from build123d import *

# Parameters (mm, degrees)
F0_W     = 3.175
F0_H     = 28.575
F1_DEPTH = 15.875
F2_R     = 3.175
F3_R     = 5.08
F4_R     = 4.7625
F5_DEPTH = 3.176
F6_W     = 4.7625
F6_H     = 11.1125
F7_DEPTH = 25.4


with BuildPart() as f1:
    # F0 (on Front) → F1 (new body, symmetric)
    with BuildSketch(Plane.XZ):
        with BuildLine():
            ThreePointArc((-160.35073, 0), (-117.864138, 109.335137), (-12.7, 161.294609))
            Line((-12.7, 161.294609), (-12.7, 211.800312))
            Line((-12.7, 211.800312), (-15.875, 211.800312))
            Line((-15.875, 211.800312), (-15.875, 164.175312))
            ThreePointArc((-15.875, 164.175312), (-121.183386, 110.401847), (-163.52573, 0))
            Line((-163.52573, 0), (-163.52573, -161.925))
            Line((-163.52573, -161.925), (-160.35073, -161.925))
            Line((-160.35073, -161.925), (-160.35073, 0))
        make_face()
        with Locations((-161.93823, -176.2125)):
            Rectangle(F0_W, F0_H)
    extrude(amount=F1_DEPTH, both=True)

    # F2
    f2_edges = [f1.edges().sort_by_distance(p)[0] for p in [
        (-15.875, 0, 164.175312),
    ]]
    fillet(f2_edges, radius=F2_R)

    # F3
    f3_edges = [f1.edges().sort_by_distance(p)[0] for p in [
        (-12.7, 0, 161.294609),
    ]]
    fillet(f3_edges, radius=F3_R)

    # F4 (on face) → F5 (cut, through all)
    with BuildSketch(Plane(origin=(-15.875, 0, 0), x_dir=(0, -1, 0), z_dir=(-1, 0, 0))):
        with Locations((0, 192.750312)):
            Circle(F4_R)
    extrude(amount=-F5_DEPTH, mode=Mode.SUBTRACT)

    # F6 (on face) → F7 (cut)
    with BuildSketch(Plane(origin=(-163.52573, 0, 0), x_dir=(0, -1, 0), z_dir=(-1, 0, 0))):
        with Locations((-13.49375, -162.71875)):
            Rectangle(F6_W, F6_H)
        with Locations((13.49375, -162.71875)):
            Rectangle(F6_W, F6_H)
    extrude(amount=-F7_DEPTH, mode=Mode.SUBTRACT)


solid = f1.part
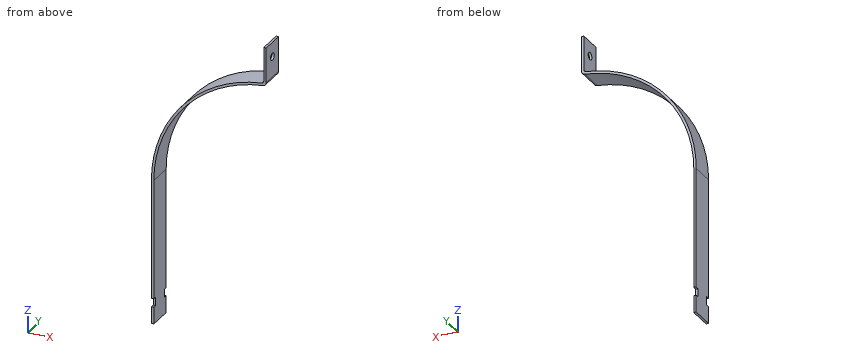
Geometry: final body of the model. Coordinates: model frame, mm. Coordinates: 2 decimals unless noted, no trailing zeros. Order: outer loops, then holes, each group sorted by start corner. A loop starts at its lowest first (then second) coordinate and runs counter-clockwise, first axis right, second up.
(1) First-contact query: pin 1 (9.5 mm diameter, centred on y = 3.5, z = 195.5, fed in from -X) (3 decimals); pin 2 (8.5 mm diameter, centred on y = 0, z = 192.75, fed in from -X); pin 3 (4 mm diameter, centred on y = -0.5, z = 119, fed in from +X); pin 4 (6 mm diameter, centred on y = -11.5, z = -68.5, fed in from +X). Flat tips, straight axial feed; report the tip coordinate or a pass-through.
(2) Section query B-B (z = -122). Return the cut outline in (x, y) (3 decimals).
(3) Section query A-A (y = 0). Return the cut outline in (x, z) (3 decimals), plus the area to 3 significant figures.
(4) Material intervals for probe 1 along X at (y, z) = (-10.5, -105); probe 2 along X at (y, z) = (-10, 2); probe 3 along Z at (x, y) = (-15.2, 0), sorted ascending.
(5) Section query C-C (x = -126.5). Return the cut outline in (y, z) (3 decimals).
Solution:
1. pin 1: stops at x = -15.875
1. pin 2: passes through
1. pin 3: stops at x = -106.03
1. pin 4: stops at x = -160.35
2. outline: (-163.526, -15.875) - (-160.351, -15.875) - (-160.351, 15.875) - (-163.526, 15.875) - close
3. outline: (-163.526, -190.5) - (-160.351, -190.5) - (-160.351, 0) arc R161.925 cw to (-17.191, 160.834) arc R5.08 ccw to (-12.7, 165.88) - (-12.7, 187.988) - (-15.875, 187.988) - (-15.875, 167.006) arc R3.175 cw to (-18.661, 163.855) arc R165.1 ccw to (-163.526, 0) - close; (-15.875, 197.513) - (-12.7, 197.513) - (-12.7, 211.8) - (-15.875, 211.8) - close
3. area: 1,490 mm2
4. probe 1: x = -163.53 to -160.35
4. probe 2: x = -163.51 to -160.34
4. probe 3: z = 161.5 to 187.99, 197.51 to 211.8
5. outline: (-15.875, 99.079) - (15.875, 99.079) - (15.875, 104.187) - (-15.875, 104.187) - close
